Build history of the part. All positions in model axes, mm. Face numbers are marked on the shaded views. A direction names the side the tool comes from. Coordinates: 2 decimals unless noted, no trailing zeros. Write each loop counter-clockwise with the first axis right and the second up, starting at its lowest first coordinate (ties: lowest second). Pieces come first, ordered by that corner, then holes. Notation, with made-up numbers: (4.25, -6) -> (9.25, -6) arc R15 ccw to (9.25, 9) -> close; hole circle Ø2 at (30, 88). An arc over 180 degrees is marked (long way). Write each question's results on one line, items separated by ' | '. Start each with the question number.
Q1. Saw through at B-B on x = 0. Give the cut face in (y, z), and give its area (3 significant figures).
Q2. Saw through at C-C on z = 6.25. Give the cut face in (x, y), and give its area (3 significant figures).
Q3. Two-plate mould, pull along X, no slides. Class the marked faces 1, 2 and 3: released by +X, released by -X, zero draft, split by the parting line, or undercut.
Q4. Drill centre lines: line 1 (Z direction, x = 0, y = -3.5); line 2 (X direction, y = -3.5, z = 10); line 3 (X direction, y = -1, z = 2). Where is each one in solid material? Low to high.
Q5. Tool access for the marked faces 4 and 5: list every direction of +Z, -Z, +X, -X, +Y, -Y with a clear straight run to the whole face (end or side of a thin tool).
Q6. Saw through at A-A on z = 10. Give the cut face in (x, y), and give its area (3 significant figures).
Q7. Drop flat-ended pins along their axis: pin 1 Ø1.5 at (x, z) = (6, 9) entering from +Y; pin 2 Ø4 at (x, z) = (0, 10) entering from +Y; pin 3 Ø5 at (y, z) = (-5.5, 6) entering from +X. Give the stop position or say it passes through.
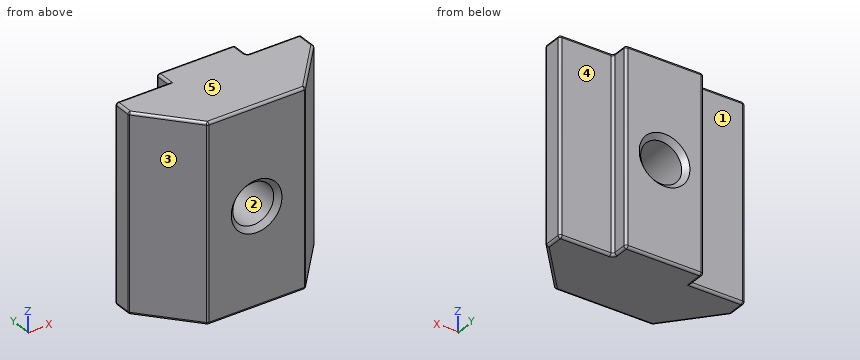
from build123d import *

# Parameters (mm, degrees)
BOSS_EXTRUDE1_DEPTH   = 20
M5X0_8_TAPPED_HOLE1_D = 4.2
CHAMFER1_SIZE         = 0.5
FILLET1_R             = 0.25


with BuildPart() as part:
    # Sketch1 → Boss-Extrude1 (new body)
    with BuildSketch(Plane.XY):
        Polygon((-4, 0), (4, 0), (4, -1.8), (9.5, -1.8), (9.5, -3.8), (5, -9), (-5, -9), (-9.5, -3.8), (-9.5, -1.8), (-4, -1.8), align=None)
    extrude(amount=BOSS_EXTRUDE1_DEPTH)

    # M5x0.8 Tapped Hole1 (through all)
    with Locations(Plane(origin=(0, 0, 0), x_dir=(1, 0, 0), z_dir=(0, 1, 0))):
        with Locations((0, -10)):
            Hole(M5X0_8_TAPPED_HOLE1_D / 2)

    # Chamfer1
    chamfer1_edges = [part.edges().sort_by_distance(p)[0] for p in [
        (2.1, 0, 10),
        (2.1, -9, 10),
    ]]
    chamfer(chamfer1_edges, length=CHAMFER1_SIZE)

    # Fillet1
    fillet1_edges = [part.edges().sort_by_distance(p)[0] for p in [
        (-4, -0.9, 20),
        (7.25, -6.4, 0),
        (0, -9, 0),
        (-7.25, -6.4, 0),
        (-9.5, -2.8, 0),
        (-6.75, -1.8, 0),
        (-4, -0.9, 0),
        (0, 0, 0),
        (4, -0.9, 0),
        (-6.75, -1.8, 20),
        (-9.5, -2.8, 20),
        (4, -1.8, 10),
        (9.5, -1.8, 10),
        (9.5, -3.8, 10),
        (5, -9, 10),
        (-5, -9, 10),
        (-9.5, -3.8, 10),
        (-9.5, -1.8, 10),
        (-4, 0, 10),
        (4, 0, 10),
        (-7.25, -6.4, 20),
        (0, -9, 20),
        (7.25, -6.4, 20),
        (9.5, -2.8, 20),
        (6.75, -1.8, 20),
        (4, -0.9, 20),
        (0, 0, 20),
        (6.75, -1.8, 0),
        (9.5, -2.8, 0),
    ]]
    fillet(fillet1_edges, radius=FILLET1_R)


solid = part.part
Returned:
1) outline: (-9, 0.25) arc R0.25 ccw to (-8.75, 0) -> (-0.25, 0) arc R0.25 ccw to (0, 0.25) -> (0, 7.4) -> (-0.5, 7.9) -> (-8.5, 7.9) -> (-9, 7.4) -> close; (-9, 12.6) -> (-8.5, 12.1) -> (-0.5, 12.1) -> (0, 12.6) -> (0, 19.75) arc R0.25 ccw to (-0.25, 20) -> (-8.75, 20) arc R0.25 ccw to (-9, 19.75) -> close | area: 142 mm2
2) outline: (-9.5, -3.71) arc R0.25 ccw to (-9.44, -3.87) -> (-5.07, -8.91) arc R0.25 ccw to (-4.89, -9) -> (4.89, -9) arc R0.25 ccw to (5.07, -8.91) -> (9.44, -3.87) arc R0.25 ccw to (9.5, -3.71) -> (9.5, -2.05) arc R0.25 ccw to (9.25, -1.8) -> (4.25, -1.8) arc R0.25 cw to (4, -1.55) -> (4, -0.25) arc R0.25 ccw to (3.75, 0) -> (-3.75, 0) arc R0.25 ccw to (-4, -0.25) -> (-4, -1.8) -> (-9.25, -1.8) arc R0.25 ccw to (-9.5, -2.05) -> close | area: 128 mm2
3) face 1: zero draft | face 2: undercut | face 3: released by -X
4) line 1: z = 0 to 7.9, 12.1 to 20 | line 2: x = -9.5 to -2.1, 2.1 to 9.5 | line 3: x = -4 to 4
5) face 4: +Z, -Z, +X, +Y | face 5: +Z, +X, -X, +Y, -Y
6) outline: (-9.5, -3.71) arc R0.25 ccw to (-9.44, -3.87) -> (-5.07, -8.91) arc R0.25 ccw to (-4.89, -9) -> (-2.6, -9) -> (-2.1, -8.5) -> (-2.1, -0.5) -> (-2.6, 0) -> (-3.75, 0) arc R0.25 ccw to (-4, -0.25) -> (-4, -1.8) -> (-9.25, -1.8) arc R0.25 ccw to (-9.5, -2.05) -> close; (2.1, -8.5) -> (2.6, -9) -> (4.89, -9) arc R0.25 ccw to (5.07, -8.91) -> (9.44, -3.87) arc R0.25 ccw to (9.5, -3.71) -> (9.5, -2.05) arc R0.25 ccw to (9.25, -1.8) -> (4.25, -1.8) arc R0.25 cw to (4, -1.55) -> (4, -0.25) arc R0.25 ccw to (3.75, 0) -> (2.6, 0) -> (2.1, -0.5) -> close | area: 89.5 mm2
7) pin 1: stops at y = -1.8 | pin 2: passes through | pin 3: stops at x = 9.5
